Here's how the part is built. I have some questions about the finished solid (model axes, mm). A direction names the side the tool comes from. Coordinates: 2 decimals unless noted, no trailing zeros. Write each loop counter-clockwise with the first axis right and the second up, starting at its lowest first coordinate (ties: lowest second). Pieces come first, ordered by that corner, then holes. Notation, with made-up numbers: (48.25, 16) -> (71.25, 16) arc R28 ccw to (71.25, 34) -> close; hole circle Ø5 at (-9.5, 53.5). An arc over 180 degrees is marked (long way). Use CSV: the item, a comma, the result in double quotes. Start each with the question number.
```python
from build123d import *

# Parameters (mm, degrees)
SKETCH1_W           = 1066.8
SKETCH1_H           = 101.6
BOSS_EXTRUDE1_DEPTH = 19.05
SKETCH2_R           = 19.05
SKETCH2_R_2         = 2.38125
BOSS_EXTRUDE2_DEPTH = 19.05
SKETCH4_R           = 19.05
CUT_EXTRUDE1_DEPTH  = 9.525


with BuildPart() as part:
    # Sketch1 → Boss-Extrude1 (new body)
    with BuildSketch(Plane.XY):
        Rectangle(SKETCH1_W, SKETCH1_H)
    extrude(amount=BOSS_EXTRUDE1_DEPTH)

    # Sketch2 → Boss-Extrude2 (add)
    # profile 1 of 3: a face of its own
    with BuildSketch(Plane.XY.offset(19.05)):
        with BuildLine():
            Line((-514.35, -50.8), (-425.45, -50.8))
            Line((-425.45, -50.8), (-425.45, -82.55))
            ThreePointArc((-425.45, -82.55), (-469.9, -127), (-514.35, -82.55))
            Line((-514.35, -82.55), (-514.35, -50.8))
        make_face()
        with Locations((-469.9, -82.55)):
            Circle(SKETCH2_R, mode=Mode.SUBTRACT)
    # profile 2 of 3: a face of its own
    with BuildSketch(Plane.XY.offset(19.05)):
        with BuildLine():
            Line((514.35, -50.8), (425.45, -50.8))
            Line((425.45, -50.8), (425.45, -82.55))
            ThreePointArc((425.45, -82.55), (469.9, -127), (514.35, -82.55))
            Line((514.35, -82.55), (514.35, -50.8))
        make_face()
        with Locations((469.9, -82.55)):
            Circle(SKETCH2_R_2, mode=Mode.SUBTRACT)
    # profile 3 of 3: a face of its own
    with BuildSketch(Plane.XY.offset(19.05)):
        with BuildLine():
            Line((-260.35, -50.8), (-171.45, -50.8))
            Line((-171.45, -50.8), (-171.45, -82.55))
            ThreePointArc((-171.45, -82.55), (-215.9, -127), (-260.35, -82.55))
            Line((-260.35, -82.55), (-260.35, -50.8))
        make_face()
        with Locations((-215.9, -82.55)):
            Circle(SKETCH2_R, mode=Mode.SUBTRACT)
    extrude(amount=-BOSS_EXTRUDE2_DEPTH)

    # Sketch4 → Cut-Extrude1 (cut)
    with BuildSketch(Plane(origin=(0, 0, 0), x_dir=(-1, 0, 0), z_dir=(0, 0, -1))):
        with Locations((-469.9, -82.55)):
            Circle(SKETCH4_R)
    extrude(amount=-CUT_EXTRUDE1_DEPTH, mode=Mode.SUBTRACT)


solid = part.part
```
Item 1: I'm going to push flat-ended pins straight in: pin 1 (5.5 mm diameter, centred on y = -65, z = 11, fed in from +X); pin 2 (5.5 mm diameter, centred on x = 528, z = 12.5, fed in from -Y); pin 3 (23 mm diameter, centred on x = -215.9, y = -82.55, fed in from -Z); pin 4 (6 mm diameter, centred on x = 469.9, y = -82.55, fed in from -Z) (3 decimals). Where does each tip first touch, or does it pass through?
Item 2: Which directions (+Z, -Z, +X, -X, +Y, -Y) give clear straight access to the entire face, cutting with the end or side of a thin tool? Please do faces 1 (the flat face through (123, -50.8, 9)), 2 (the flat face through (514.35, -67, 10)), 3 (the cylindrical face through (-234.93, -81.71, 9.66)), 4 (the cylindrical face through (488.93, -81.71, 4.7)).
Item 3: I want a section at C-C on z = 6.25. Please give me the cut outline in (x, y).
Item 4: I want a section at A-A on x = -469.9. Please give me the cut outline in (y, z), then the cut area to 3 significant figures.
Item 5: Thinking about a two-plate mould opening in X: for faces 5 (the cylindrical face through (468.92, -126.99, 9.66)), 6 (the flat face through (533.4, -1, 9)), 7 (the flat face through (-7, -17, 19.05)), which applies, +X half, -X half, draft (parallel to the pull), parting line (faces both ways), or undercut?
Item 6: I want a section at D-D on x = 290. Please give me the cut outline in (y, z), then the cut area to 3 significant figures.
Item 7: I want a section at B-B on y = -111. Please give me the cut outline in (x, z).
Item 8: If I drill on line 1 along X through (y, z) = (-60.5, 5.5); line 2 along Y through (x, z) = (-215.9, 15.25); line 3 along Y through (x, z) = (469.9, 16), over which ranges is the centre line in solid material (lowest first)?
Geometry says:
1,pin 1,"x = 514.35"
1,pin 2,"y = -50.8"
1,pin 3,"through"
1,pin 4,"z = 9.525"
2,face 1,"+Z, -Z, -Y"
2,face 2,"+Z, -Z, +X, -Y"
2,face 3,"+Z, -Z"
2,face 4,"-Z"
3,outline,"(-533.4, -50.8) -> (-514.35, -50.8) -> (-514.35, -82.55) arc R44.45 ccw to (-425.45, -82.55) -> (-425.45, -50.8) -> (-260.35, -50.8) -> (-260.35, -82.55) arc R44.45 ccw to (-171.45, -82.55) -> (-171.45, -50.8) -> (425.45, -50.8) -> (425.45, -82.55) arc R44.45 ccw to (514.35, -82.55) -> (514.35, -50.8) -> (533.4, -50.8) -> (533.4, 50.8) -> (-533.4, 50.8) -> close; hole circle Ø38.1 at (-469.9, -82.55); hole circle Ø38.1 at (-215.9, -82.55); hole circle Ø38.1 at (469.9, -82.55)"
4,outline,"(-127, 0) -> (-101.6, 0) -> (-101.6, 19.05) -> (-127, 19.05) -> close; (-63.5, 0) -> (50.8, 0) -> (50.8, 19.05) -> (-63.5, 19.05) -> close"
4,area,"2,660 mm2"
5,face 5,"undercut"
5,face 6,"+X half"
5,face 7,"draft"
6,outline,"(-50.8, 0) -> (50.8, 0) -> (50.8, 19.05) -> (-50.8, 19.05) -> close"
6,area,"1,940 mm2"
7,outline,"(-504.05, 0) -> (-435.75, 0) -> (-435.75, 19.05) -> (-504.05, 19.05) -> close; (-250.05, 0) -> (-181.75, 0) -> (-181.75, 19.05) -> (-250.05, 19.05) -> close; (435.75, 0) -> (504.05, 0) -> (504.05, 19.05) -> (435.75, 19.05) -> close"
8,line 1,"-514.35 to -425.45, -260.35 to -171.45, 425.45 to 514.35"
8,line 2,"-127 to -101.6, -63.5 to 50.8"
8,line 3,"-127 to -84.93, -80.17 to 50.8"
